Design review of the part built by this model. Coordinates are the model's own, in mm. Face numbers are marked on the shaded views. A direction names the side the tool comes from. Give positions to 0.01 mm unless a question says otherwise; leave off trailing zeros. Loops run counter-clockwise (first coordinate to the right, second up) from the corner with the lowest first, then second, coordinate; pieces in that order, holes last. Notation, with made-up numbers: M -15,80.5 L 33,80.5 A15 ccw 33,106.5 Z; hole C 46,22 d2. An arc over 180 degrees is marked long. Use a Markdown table: item, result. Add a question column.
(1) Insertion check: pin 1 Ø5 at (x, z) = (32, -1) entering from -Y; pin 2 Ø5.5 at (x, z) = (76, -0.5) entering from -Y; pin 3 Ø1 at (y, z) = (7, 6) entering from +X. Each pin has a flat end and moves straight along its axis. Give the tip position at first contact, or say it passes through.
(2) Add section D-D, the plane x = -6. Give the boundary of the cut face in (y, z).
(3) For the marked faces 1 and 2, list the 3-axis set-ups (+Z, -Z, +X, -X, +Y, -Y) from which the entire face can be reached by the end or side of a thin tool; tool diameter is ignored.
(4) Add section C-C, the plane y = 8. Give the boundary of the cut face in (x, z), then the cut area to 3 significant figures.
(5) For probe 1 along X at (y, z) = (3, -5.08); probe 2 along X at (y, z) = (-10, 7.62); probe 3 along X at (y, z) = (-15, -0.5), list the stretches that pass through material, from the lowest coordinate up.
(6) Add section B-B, the plane z = -5.08. Give the boundary of the cut face in (x, y), then the cut area to 3 significant figures.
(7) Add section A-A, the plane y = -12.5. Give the boundary of the cut face in (x, z), then the cut area to 3 significant figures.
(8) Draft analysis for pull direction X (two halves, no side actions). For the marked faces 3, 4, 5 and 6, state which applies: pulls with the +X half, pulls with the -X half, needs draft (parallel to the pull), parting line crosses it, or undercut.
```python
from build123d import *

# Parameters (mm, degrees)
BOSS_EXTRUDE1_DEPTH      = 13.97
BOSS_EXTRUDE1_DEPTH_BACK = 10.16
SKETCH1_W                = 11.43
SKETCH1_H                = 17.78
SKETCH1_W_2              = 152.4
SKETCH1_H_2              = 12.7
SKETCH1_H_3              = 16.41011236
CHAMFER1_SIZE            = 6.35
SKETCH2_R                = 3.048
SKETCH2_R_2              = 3.190843713
SKETCH2_R_3              = 3.125749827
CUT_EXTRUDE1_DEPTH       = 88.976767749
CHAMFER2_SIZE            = 3.81


with BuildPart() as part:
    # Sketch1 → Boss-Extrude1 (new, two sides: drawn at the far end of the back side and taken through both)
    with BuildSketch(Plane.XY.offset(-BOSS_EXTRUDE1_DEPTH_BACK)):
        with Locations((-65.347921348, -8.89)):
            Rectangle(SKETCH1_W, SKETCH1_H)
        with Locations((5.137078652, 6.35)):
            Rectangle(SKETCH1_W_2, SKETCH1_H_2)
        with Locations((75.622078652, -8.20505618)):
            Rectangle(SKETCH1_W, SKETCH1_H_3)
    extrude(amount=BOSS_EXTRUDE1_DEPTH + BOSS_EXTRUDE1_DEPTH_BACK)

    # Chamfer1
    chamfer1_edges = [part.edges().sort_by_distance(p)[0] for p in [
        (-71.062921348, 12.7, 1.905),
        (81.337078652, 12.7, 1.905),
        (69.907078652, 0, 1.905),
        (-59.632921348, 0, 1.905),
    ]]
    chamfer(chamfer1_edges, length=CHAMFER1_SIZE)

    # Sketch2 → Cut-Extrude1 (cut, through all)
    with BuildSketch(Plane.XZ.offset(17.78)):
        with Locations((-64.865321348, 7.605218814)):
            Circle(SKETCH2_R)
        with Locations((-64.865321348, -5.08)):
            Circle(SKETCH2_R)
        with Locations(Location((76.257078652, 7.62, 0), (0, 0, 113.454073409))):
            Circle(SKETCH2_R_2)
        with Locations(Location((76.257078652, -5.08, 0), (0, 0, 113.972774897))):
            Circle(SKETCH2_R_3)
    extrude(amount=-CUT_EXTRUDE1_DEPTH, mode=Mode.SUBTRACT)

    # Chamfer2
    chamfer2_edges = [part.edges().sort_by_distance(p)[0] for p in [
        (5.137078652, 0, 13.97),
        (5.137078652, 0, -10.16),
    ]]
    chamfer(chamfer2_edges, length=CHAMFER2_SIZE)


solid = part.part
```
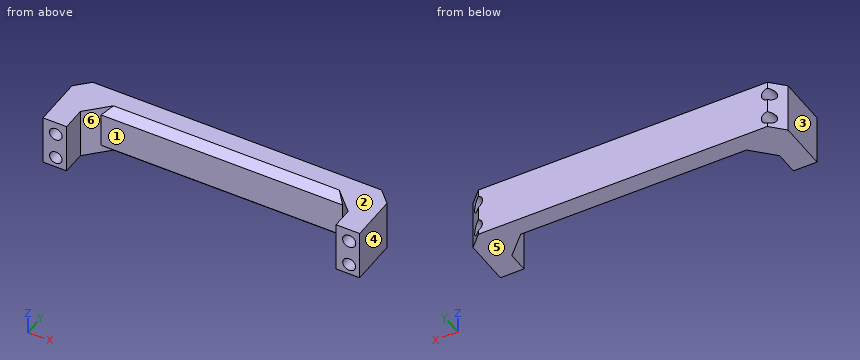
Established:
| question | item | result |
|---|---|---|
| 1 | pin 1 | y = 0 |
| 1 | pin 2 | y = -16.41 |
| 1 | pin 3 | x = 81.19 |
| 2 | outline | M 0,-6.35 L 3.81,-10.16 L 12.7,-10.16 L 12.7,13.97 L 3.81,13.97 L 0,10.16 Z |
| 3 | face 1 | +Z, -Z, -Y |
| 3 | face 2 | +Z, +X, -X, +Y, -Y |
| 4 | outline | M -69.41,-10.16 L 79.69,-10.16 L 79.69,13.97 L -69.41,13.97 Z; hole C -64.87,-5.08 d6.1; hole C -64.87,7.61 d6.1; hole C 76.26,7.62 d6.38; hole C 76.26,-5.08 d6.25 |
| 4 | area | 3,480 mm^2 |
| 5 | probe 1 | -71.06 to -67.91, -61.82 to 73.13, 79.38 to 81.34 |
| 5 | probe 2 | -71.06 to -67.91, -61.82 to -59.63, 69.91 to 73.07, 79.45 to 81.34 |
| 5 | probe 3 | -71.06 to -59.63, 69.91 to 81.34 |
| 6 | outline | M -71.06,-17.78 L -67.91,-17.78 L -67.91,9.5 L -71.06,6.35 Z; M -61.82,-17.78 L -59.63,-17.78 L -59.63,-6.35 L -53.28,0 L 63.56,0 L 69.91,-6.35 L 69.91,-16.41 L 73.13,-16.41 L 73.13,12.7 L -61.82,12.7 Z; M 79.38,-16.41 L 81.34,-16.41 L 81.34,6.35 L 79.38,8.3 Z |
| 6 | area | 1,970 mm^2 |
| 7 | outline | M -71.06,-10.16 L -59.63,-10.16 L -59.63,13.97 L -71.06,13.97 Z; M 69.91,-10.16 L 81.34,-10.16 L 81.34,13.97 L 69.91,13.97 Z; hole C -64.87,-5.08 d6.1; hole C -64.87,7.61 d6.1; hole C 76.26,7.62 d6.38; hole C 76.26,-5.08 d6.25 |
| 7 | area | 431 mm^2 |
| 8 | face 3 | pulls with the -X half |
| 8 | face 4 | pulls with the +X half |
| 8 | face 5 | needs draft |
| 8 | face 6 | undercut |
